Part print with two shaded views. Sizes in mm from the minimum x, y, z corner. Give positions to 0.01 mm unless a question says otherwise; leave off trailing zeros. Write each loop counter-clockwise with the first axis right and the second up, starting at its lowest first coordinate (ties: lowest second). Pieces come first, ordered by that corner, then holes. Notation, with made-up numbers: (-8.5, -15) - (-1.5, -15) arc R22 cw to (-1.5, 3) - close; hole circle Ø3 at (-6, -26.5). An arc over 180 degrees is marked (long way). Answer as a JSON object with one key per item and string values.
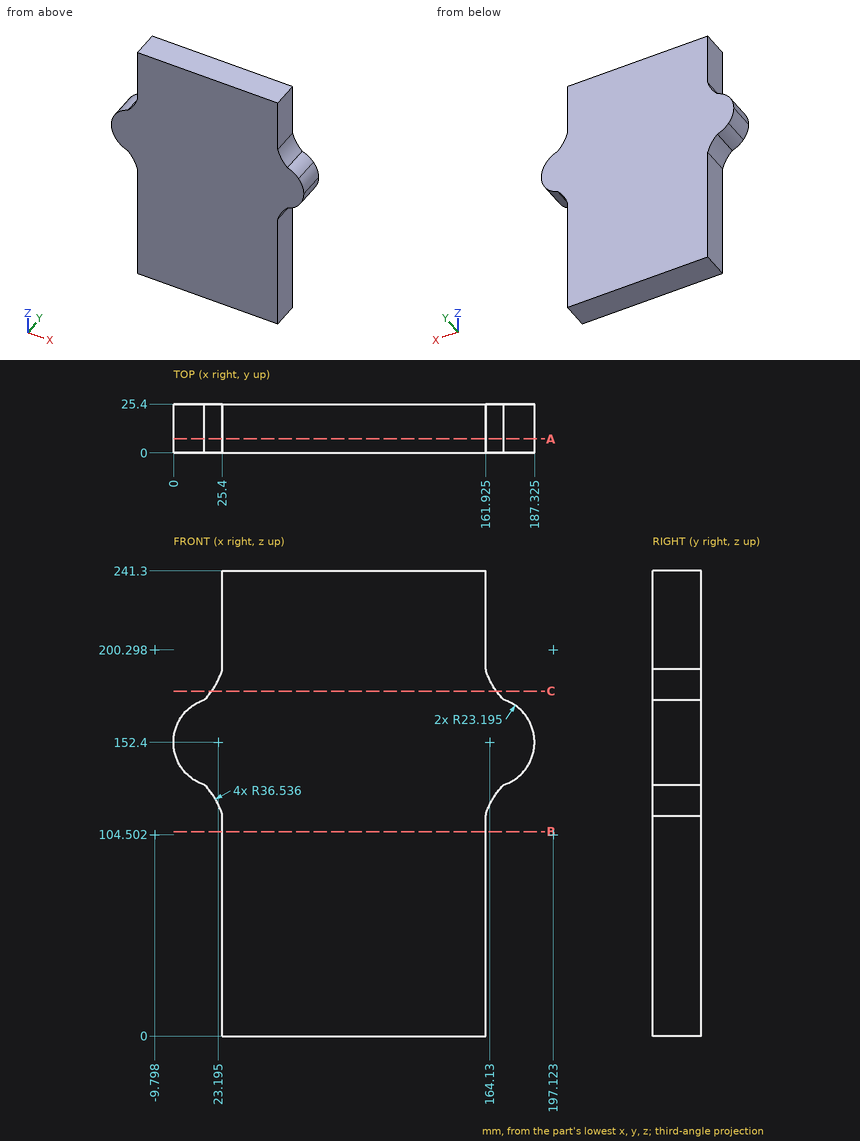
(1) Saw through at A-A, the plane y = 7.25. Give the cut face in (x, z) (1 decimal), and give its area (3 significant figures).
Answer key:
{"outline": "(16, 130.3) arc R36.5 cw to (25.4, 114.3) - (25.4, 0) - (161.9, 0) - (161.9, 114.3) arc R36.5 cw to (171.3, 130.3) arc R23.2 ccw to (171.3, 174.5) arc R36.5 cw to (161.9, 190.5) - (161.9, 241.3) - (25.4, 241.3) - (25.4, 190.5) arc R36.5 cw to (16, 174.5) arc R23.2 ccw to start", "area": "35,000 mm²"}
(2) Flat gauge pins, fed straight in: P1, Ø7.5, axis at y = 18.5, z = 203.5, coming from the +X side (3 decimals); P2, Ø8, axis at x = 60.5, y = 5, coming from the -Z side; P3, Ø4, axis at y = 21, z = 167.5, coming from the +X side; P4, Ø6, axis at y = 21.5, z = 72, coming from the -X side. Where does each tip first touch, or does it go through?
Answer key:
{"P1": "stops at x = 161.925", "P2": "stops at z = 0", "P3": "stops at x = 183.27", "P4": "stops at x = 25.4"}
(3) Saw through at B-B, the plane z = 106. Give the cut face in (x, y) (3 decimals).
Answer key:
{"outline": "(25.4, 0) - (161.925, 0) - (161.925, 25.4) - (25.4, 25.4) - close"}
(4) Probe L1, parallel to X at y = 23.5, z = 86.5 (3 decimals); L2, parallel to X at y = 8.75, z = 169 (1 decimal). List the from-to ranges inside material, lowest first. Write a range as [from, to].
Answer key:
{"L1": "x = [25.4, 161.925]", "L2": "x = [7, 180.3]"}
(5) Saw through at C-C, the plane z = 179. Give the cut face in (x, y).
Answer key:
{"outline": "(19.89, 0) - (167.44, 0) - (167.44, 25.4) - (19.89, 25.4) - close"}
